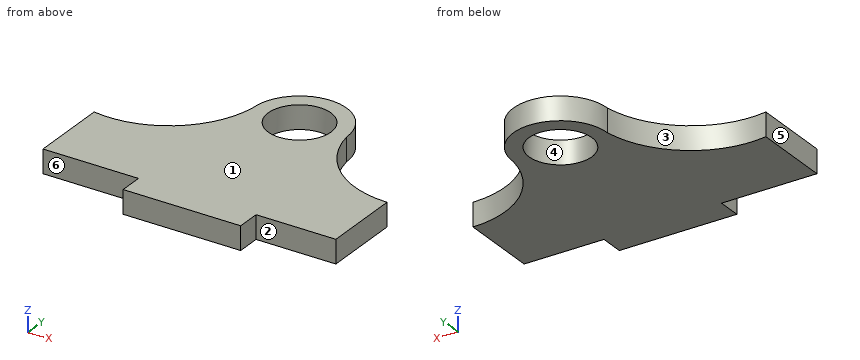
from build123d import *

# Parameters (mm, degrees)
SKETCH1_R           = 4
BOSS_EXTRUDE1_DEPTH = 3


with BuildPart() as part:
    # Sketch1 → Boss-Extrude1 (new body)
    with BuildSketch(Plane.XY):
        with BuildLine():
            Line((7.5, -20), (17.681043382, -20))
            Line((17.681043382, -20), (17.681043382, -10))
            ThreePointArc((17.681043382, -10), (9.992620207, -7.15854174), (6, 0))
            ThreePointArc((6, 0), (0, 6), (-6, 0))
            ThreePointArc((-6, 0), (-10.729319879, -7.888344359), (-19.681043382, -10))
            Line((-19.681043382, -10), (-19.681043382, -20))
            Line((-19.681043382, -20), (-7.5, -20))
            Line((-7.5, -20), (-7.5, -23))
            Line((-7.5, -23), (7.5, -23))
            Line((7.5, -23), (7.5, -20))
        make_face()
        Circle(SKETCH1_R, mode=Mode.SUBTRACT)
    extrude(amount=BOSS_EXTRUDE1_DEPTH)


solid = part.part
Source: CAD feature listing. Evaluate the final solid. Frame: model axes, mm. Face numbers are marked on the shaded views. A direction names the side the tool comes from. Coordinates: 2 decimals unless noted, no trailing zeros. Write each loop counter-clockwise with the first axis right and the second up, starting at its lowest first coordinate (ties: lowest second). Pieces come first, ordered by that corner, then holes. Notation, with made-up numbers: M -27,29 L 13,29 A14 ccw 13,46 Z; hole C 82.25,-9.75 d7. An arc over 180 degrees is marked long. Use a Markdown table: item, result.
1) Section D-D, the plane y = -5.25. Output: boundary loops of the cut face in (x, z), then the cut area to 3 significant figures.
Conclusion:
| item | result |
|---|---|
| outline | M -8.11,0 L 8.21,0 L 8.21,3 L -8.11,3 Z |
| area | 49.0 mm^2 |
2) Mould query, pull axis Y, two halves, no side actions, for the marked faces 1, 2, 3 and 4. Classes: pulls with the +Y half, pulls with the -Y half, needs draft (parallel to the pull), parting line crosses it, or undercut.
Conclusion:
| item | result |
|---|---|
| face 1 | needs draft |
| face 2 | pulls with the -Y half |
| face 3 | pulls with the +Y half |
| face 4 | undercut |
3) Section C-C, the plane x = 13. Output: boundary loops of the cut face in (y, z), then the cut area to 3 significant figures.
Conclusion:
| item | result |
|---|---|
| outline | M -20,0 L -9.03,0 L -9.03,3 L -20,3 Z |
| area | 32.9 mm^2 |
4) Section B-B, the plane x = 0. Output: boundary loops of the cut face in (y, z).
Conclusion:
| item | result |
|---|---|
| outline | M -23,0 L -4,0 L -4,3 L -23,3 Z; M 4,0 L 6,0 L 6,3 L 4,3 Z |
5) Ray query, L1, parallel to Y at x = 0, z = 1.65; L2, parallel to X at y = 0.25, z = 2.85; L3, parallel to Y at x = -1.5, z = 2.15. Return the intervals inside material, ascending.
Conclusion:
| item | result |
|---|---|
| L1 | y = -23 to -4, 4 to 6 |
| L2 | x = -5.99 to -3.99, 3.99 to 5.99 |
| L3 | y = -23 to -3.71, 3.71 to 5.81 |
6) Section A-A, the plane z = 2.5. Output: boundary loops of the cut face in (x, y).
Conclusion:
| item | result |
|---|---|
| outline | M -19.68,-20 L -7.5,-20 L -7.5,-23 L 7.5,-23 L 7.5,-20 L 17.68,-20 L 17.68,-10 A11.82 cw 6,0 A6 ccw -6,0 A11.82 cw -19.68,-10 Z; hole C 0,0 d8 |
7) Reachability of the marked faces 5 and 6 from +Z, -Z, +X, -X, +Y, -Y: full face, straight path, thin tool, end or side. Return the list, or none.
Conclusion:
| item | result |
|---|---|
| face 5 | +Z, -Z, -X, +Y, -Y |
| face 6 | +Z, -Z, -X, -Y |
8) First-contact query: pin 1 Ø1.5 at (y, z) = (-22, 2) entering from -X; pin 2 Ø3 at (x, y) = (-6.5, -5) entering from -Z. Flat tips, straight axial feed; report the tip coordinate or a pass-through.
Conclusion:
| item | result |
|---|---|
| pin 1 | stops at x = -7.5 |
| pin 2 | stops at z = 0 |
